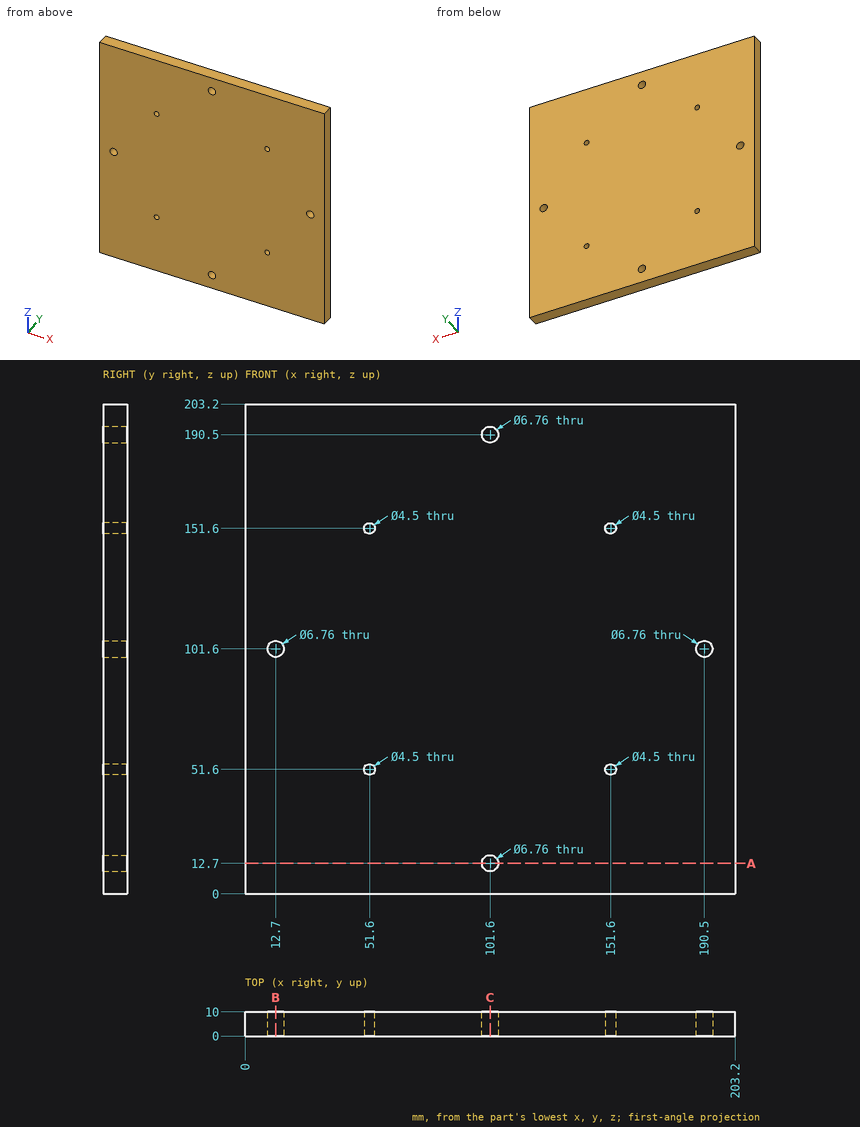
Design review of the part shown in the three views and the two pictorial views. Dimensions are in mm from the part's minimum x, y and z. Round coordinates to 2 decimals unless told otherwise and drop trailing zeros. Write each loop counter-clockwise with the first axis right and the second up, starting at its lowest first coordinate (ties: lowest second). Pieces come first, ordered by that corner, then holes.
1) Take a section at C-C on x = 101.6. Give the boundary of the cut face in (y, z), then the cut area to 3 significant figures.
Answer below:
outline: (0, 0) - (10, 0) - (10, 9.32) - (0, 9.32) - close; (0, 16.08) - (10, 16.08) - (10, 187.12) - (0, 187.12) - close; (0, 193.88) - (10, 193.88) - (10, 203.2) - (0, 203.2) - close
area: 1,900 mm2
2) Take a section at B-B on x = 12.7. Give the boundary of the cut face in (y, z), then the cut area to 3 significant figures.
Answer below:
outline: (0, 0) - (10, 0) - (10, 98.22) - (0, 98.22) - close; (0, 104.98) - (10, 104.98) - (10, 203.2) - (0, 203.2) - close
area: 1,960 mm2
3) Insertion check: pin 1 Ø2 at (x, z) = (104.5, 35) entering from -Y; pin 2 Ø6 at (x, z) = (101.6, 190.5) entering from +Y. Each pin has a flat end and moves straight along its axis. Give the tip position at first contact, or say it passes through.
Answer below:
pin 1: stops at y = 0
pin 2: passes through
4) Take a section at A-A on z = 12.7. Give the boundary of the cut face in (x, y).
Answer below:
outline: (0, 0) - (98.22, 0) - (98.22, 10) - (0, 10) - close; (104.98, 0) - (203.2, 0) - (203.2, 10) - (104.98, 10) - close
5) For line 1 along Z through (x, y) = (151.6, 7); line 2 along X through (y, z) = (2, 12.7), list the stretches that pass through material, from the lowest coordinate up.
Answer below:
line 1: z = 0 to 49.35, 53.85 to 149.35, 153.85 to 203.2
line 2: x = 0 to 98.22, 104.98 to 203.2
